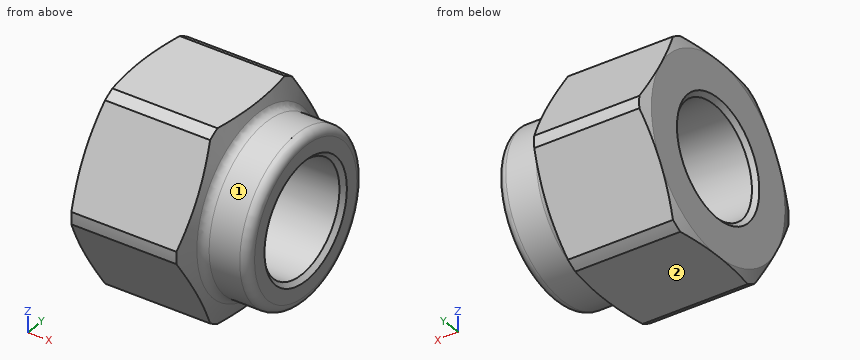
```python
from build123d import *

# Parameters (mm, degrees)
BOSS_EXTRUDE1_DEPTH = 9.525
FILLET1_R           = 0.508


with BuildPart() as part:
    # Sketch1 → Boss-Extrude1 (new body)
    with BuildSketch(Plane(origin=(0, 0, 0), x_dir=(0, 0, -1), z_dir=(1, 0, 0))):
        Polygon((0, 6.415804866), (-5.55625, 3.207902433), (-5.55625, -3.207902433), (0, -6.415804866), (5.55625, -3.207902433), (5.55625, 3.207902433), align=None)
    extrude(amount=BOSS_EXTRUDE1_DEPTH)

    # Sketch2 → Cut-Revolve2 (revolve, cut)
    with BuildSketch(Plane.XY):
        Polygon((0, 0), (9.525, 0), (9.525, 3.429), (9.271, 3.175), (0.254, 3.175), (0, 3.429), align=None)
        Polygon((0, 5.55625), (0.242677154, 6.223), (6.35, 6.223), (6.881578527, 4.7625), (9.525, 4.7625), (9.525, 6.415804866), (0, 6.415804866), align=None)
    revolve(axis=Axis((0, 0, 0), (1, 0, 0)), mode=Mode.SUBTRACT)

    # Fillet1
    fillet1_edges = [part.edges().sort_by_distance(p)[0] for p in [
        (9.525, -4.7625, 0),
        (6.881578527, -4.7625, 0),
    ]]
    fillet(fillet1_edges, radius=FILLET1_R)


solid = part.part
```
The listing builds one solid part. Answer for the finished solid, in the listing's coordinates (mm). Face numbers are marked on the shaded views. A direction names the side the tool comes from. Give positions to 0.01 mm unless a question says otherwise; leave off trailing zeros. Loops run counter-clockwise (first coordinate to the right, second up) from the corner with the lowest first, then second, coordinate; pieces in that order, holes last. Notation, with made-up numbers: M 9.25,11.5 L 19.25,11.5 A14 ccw 19.25,27.5 Z; hole C 19.25,58.25 d5. An arc over 180 degrees is marked long. One line per item, written item: value.
Q1. A cutting plane is placed at A-A on x = 4.5. Determine the outline of the cut face in (y, z) (3 decimals).
Working result:
outline: M -6.213,-0.351 L -3.411,-5.205 A6.223 ccw -2.802,-5.556 L 2.802,-5.556 A6.223 ccw 3.411,-5.205 L 6.213,-0.351 A6.223 ccw 6.213,0.351 L 3.411,5.205 A6.223 ccw 2.802,5.556 L -2.802,5.556 A6.223 ccw -3.411,5.205 L -6.213,0.351 A6.223 ccw Z; hole C 0,0 d6.35
Q2. For the marked faces 1 and 2, determine the directions among +Z, -Z, +X, -X, +Y, -Y from which every point of the face is accessible in a straight line to the end or side of a thin tool.
Working result:
face 1: +X
face 2: -Z, +X, -X, +Y, -Y
Q3. Find the intervals of material crossed by line 1 (Z direction, x = 5.5, y = 0) (3 decimals); line 2 (Z direction, x = 8, y = 0) (1 decimal); line 3 (Y direction, x = 0.75, z = 1.25), in increasing order. Write a range as from..to.
Working result:
line 1: z = -5.556..-3.175, 3.175..5.556
line 2: z = -4.8..-3.2, 3.2..4.8
line 3: y = -5.69..-2.92, 2.92..5.69
Q4. Flat-ended cylindrical pins translate along their axes: P1, Ø1.5, axis at x = 6, z = 2.5, coming from the +Y side; P2, Ø2, axis at x = 8, y = -1, coming from the +Z side. Find the tip coordinate at first contact, or state that the pin passes through.
Working result:
P1: stops at y = 5.41
P2: stops at z = 4.76
